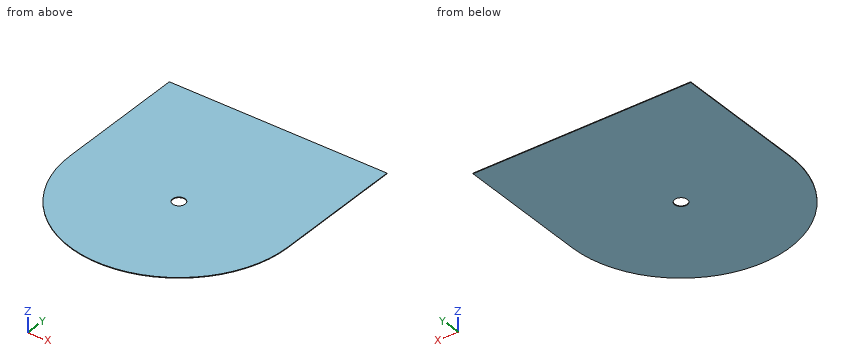
from build123d import *

# Parameters (mm, degrees)
SKETCH1_R           = 20
BOSS_EXTRUDE1_DEPTH = 2


with BuildPart() as part:
    # Sketch1 → Boss-Extrude1 (new body)
    # profile 1 of 2: a face of its own
    with BuildSketch(Plane.XY):
        with BuildLine():
            Line((-375.902130633, 412.038787591), (-375.902130633, -7.061212409))
            ThreePointArc((-375.902130633, -7.061212409), (-31.002130633, -351.961212409), (313.897869367, -7.061212409))
            Line((313.897869367, -7.061212409), (313.897869367, 412.038787591))
            Line((313.897869367, 412.038787591), (311.897869367, 412.038787591))
            Line((311.897869367, 412.038787591), (311.897869367, -7.061212409))
            ThreePointArc((311.897869367, -7.061212409), (-31.002130633, -349.961212409), (-373.902130633, -7.061212409))
            Line((-373.902130633, -7.061212409), (-373.902130633, 412.038787591))
            Line((-373.902130633, 412.038787591), (-375.902130633, 412.038787591))
        make_face()
    # profile 2 of 2: a face of its own
    with BuildSketch(Plane.XY):
        with BuildLine():
            Line((311.897869367, 412.038787591), (-373.902130633, 412.038787591))
            Line((-373.902130633, 412.038787591), (-373.902130633, -7.061212409))
            ThreePointArc((-373.902130633, -7.061212409), (-31.002130633, -349.961212409), (311.897869367, -7.061212409))
            Line((311.897869367, -7.061212409), (311.897869367, 412.038787591))
        make_face()
        with Locations((-31.002130633, -7.061212409)):
            Circle(SKETCH1_R, mode=Mode.SUBTRACT)
    extrude(amount=BOSS_EXTRUDE1_DEPTH)


solid = part.part
Here's how the part is built. I have some questions about the finished solid (model axes, mm). Give positions to 0.01 mm unless a question says otherwise; leave off trailing zeros. Order: outer loops, then holes, each group sorted by start corner. A loop starts at its lowest first (then second) coordinate and runs counter-clockwise, first axis right, second up. Notation, with made-up numbers: (27.5, -16.5) -> (71.5, -16.5) arc R30 ccw to (71.5, 7.5) -> close; hole circle Ø7 at (15, 71). An arc over 180 degrees is marked (long way). Use a Markdown table: item, result. Add a question column.
Item 1: I need wall thicknesses on line 1 (Y direction, x = -36, z = 1.2) (3 decimals); line 2 (X direction, y = -126, z = 0.9); line 3 (Y direction, x = -86.5, z = 0.4). Which ranges of each line are inside material? Lowest first, please.
Item 2: Imagine slicing it at C-C on y = -174. Please give me the cut outline in (x, z).
Item 3: Imagine slicing it at A-A on z = 0.45. Please give me the cut outline in (x, y).
Item 4: Will these pins go through, and if not, where does the flat tip stop? pin 1 (1 mm diameter, centred on x = -207, z = 1.5, fed in from -Y); pin 2 (1 mm diameter, centred on y = -263, z = 1.5, fed in from -X).
Item 5: Imagine slicing it at B-B on x = -268.5. Please give me the cut outline in (y, z).
Data:
| question | item | result |
|---|---|---|
| 1 | line 1 | y = -351.925 to -26.427, 12.304 to 412.039 |
| 1 | line 2 | x = -354.75 to 292.74 |
| 1 | line 3 | y = -347.47 to 412.04 |
| 2 | outline | (-332.81, 0) -> (270.8, 0) -> (270.8, 2) -> (-332.81, 2) -> close |
| 3 | outline | (-375.9, -7.06) arc R344.9 ccw to (313.9, -7.06) -> (313.9, 412.04) -> (-375.9, 412.04) -> close; hole circle Ø40 at (-31, -7.06) |
| 4 | pin 1 | stops at y = -303.97 |
| 4 | pin 2 | stops at x = -262.75 |
| 5 | outline | (-257.16, 0) -> (412.04, 0) -> (412.04, 2) -> (-257.16, 2) -> close |
